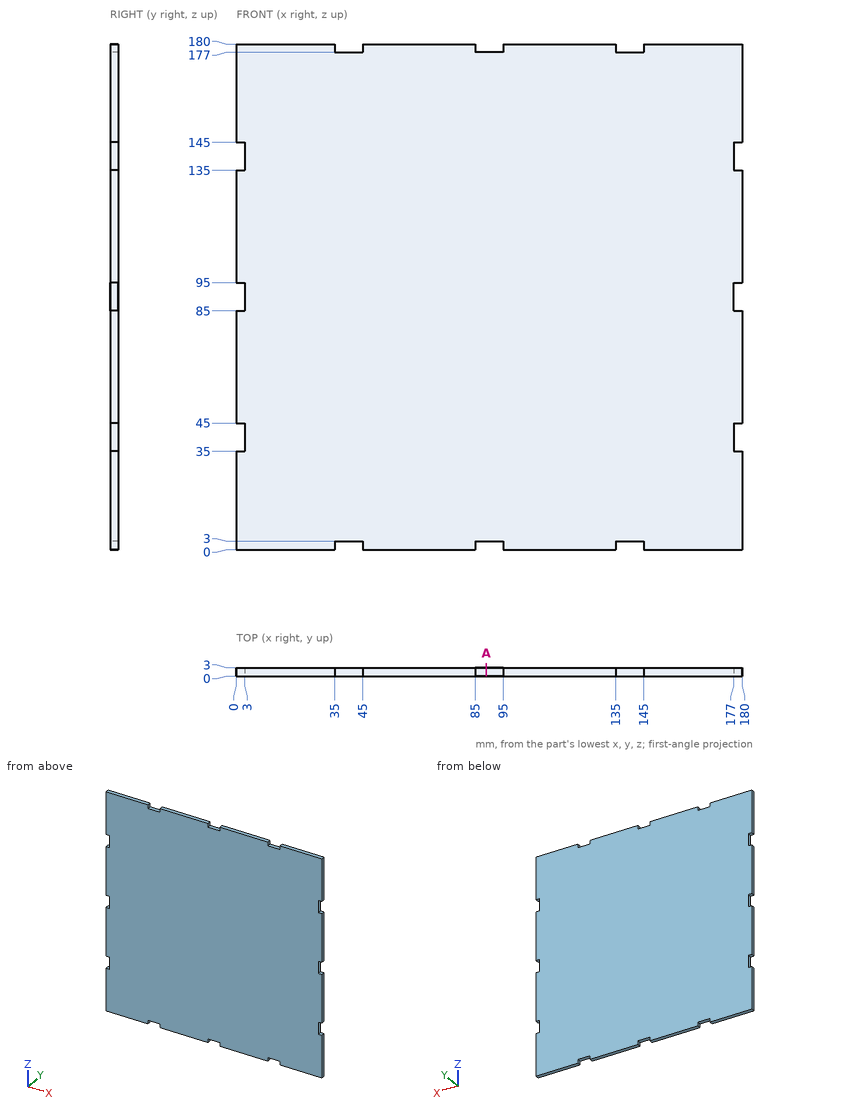
Design review of the part shown in the three views and the two pictorial views. Dimensions are in mm from the part's minimum x, y and z. Round coordinates to 2 decimals unless told otherwise and drop trailing zeros. Loops run counter-clockwise (first coordinate to the right, second up) from the corner with the lowest first, then second, coordinate; pieces in that order, holes last. Notation, with made-up numbers: (-4.5, -37.5) -> (9.5, -37.5) arc R30 ccw to (9.5, 0.5) -> close; hole circle Ø1 at (-34.75, 0.25). An arc over 180 degrees is marked (long way). Answer as a JSON object with one key per item and string values. Group by question number.
1) We need section A-A on x = 89. Write out the cut boundary in (y, z).
2) For line 1 (X direction, y = 1.2, z = 39.5), list the stretches that pass through material, from the lowest coordinate up. Write a range as [from, to].
3) For pin 1 Ø0.9 at (y, z) = (1, 179) entering from -X; pin 2 Ø0.9 at (x, y) = (41, 2) entering from +Z; pin 3 Ø0.9 at (y, z) = (2, 89.5) entering from +X, all flat-tipped, find the tip position at first contact; note any pin that passes through.
Result set:
{
 "1": {"outline": "(0, 3) -> (3, 3) -> (3, 177) -> (0, 177) -> close"},
 "2": {"line 1": "[3, 177]"},
 "3": {"pin 1": "x = 0", "pin 2": "z = 177", "pin 3": "x = 177"}
}
